Check sheet for the modelled part. Datum: model origin and axes. Units: mm. A direction names the side the tool comes from. Coordinates: 2 decimals unless noted, no trailing zeros. Write each loop counter-clockwise with the first axis right and the second up, starting at its lowest first coordinate (ties: lowest second). Pieces come first, ordered by that corner, then holes. Notation, with made-up numbers: (79.25, -1.75) - (113.25, -1.75) arc R8 ccw to (113.25, 6.25) - close; hole circle Ø9 at (-36.75, 3.5). An arc over 180 degrees is marked (long way). Answer as CSV lines item,"result". Start each with the question number.
Autodesk Inventor part; units mm, degrees
ref_plane "YZ Plane" through (0, 0, 0) normal (1, 0, 0) x (0, 1, 0)
ref_plane "XZ Plane" through (0, 0, 0) normal (0, 1, 0) x (-1, 0, 0)
ref_plane "XY Plane" through (0, 0, 0) normal (0, 0, 1) x (1, 0, 0)
sketch "Sketch4" plane through (0, 0, 0) normal (0, 1, 0) x (-1, 0, 0)
  line L0 (20, -35) -> (-20, -35)
  line L1 (-20, -35) -> (-20, 0)
  line L2 (-20, 0) -> (20, 0)
  line L3 (20, 0) -> (20, -35)
  point P0 (0, 0)
  point P1 (0, 0)
  dimension "d36" = 40
  dimension "d37" = 35
extrude "Plate2" add sketch "Sketch4" along normal blind 3
sketch "Sketch5" plane through (0, 0, 0) normal (0, -1, 0) x (1, 0, 0)
  circle A0 centre (0, -20) radius 6.5
  line L0 (0, 0) -> (0, -35) construction
  line L1 (20, -35) -> (-20, -35) construction
  dimension "d40" = 15
  dimension "d41" = 13
extrude "Cut1" cut sketch "Sketch5" against normal blind 3
sketch "Sketch6" plane through (-20, 3, -3) normal (0, 0, 1) x (1, 0, 0)
  line L0 (40, 0) -> (0, 0)
  line L1 (0, 0) -> (0, -40)
  line L2 (0, -40) -> (40, -40)
  line L3 (40, -40) -> (40, 0)
edge flange "Flange1" height 40 angle 90 thickness 3 bend radius 5 thickness toward (0, 0, 1) relief round relief width 3 relief depth 1.5 edges at (0, 0, 0) wall of the first edge with corners at (20, 3, -3) (-20, 3, -3) (-20, -37, -3) (20, -37, -3)
bend "Bend1"
corner "Corner1"
fillet "Corner Round6" radius 6 4 edges at (20, -37, -1.5) (-20, 1.5, -35) (20, 1.5, -35) (-20, -37, -1.5)
equation "\"d42\" = Thickness"
equation "\"d38\" = Thickness"
equation "\"d44\" = BendReliefWidth"
equation "\"d45\" = BendReliefDepth"
equation "\"d46\" = MinimumRemnant"
equation "\"d47\" = TransitionRadius"
equation "\"d50\" = BendRadius"
equation "\"d51\" = CornerReliefSize"
equation "\"d52\" = GapSize"
equation "\"d53\" = JacobiRadiusSize"
equation "\"BendReliefWidth\" = Thickness"
equation "\"BendReliefDepth\" = 0.5 * Thickness"
equation "\"CornerReliefSize\" = 4 * Thickness"
equation "\"MinimumRemnant\" = 2 * Thickness"
equation "\"TransitionRadius\" = BendRadius"
equation "\"JacobiRadiusSize\" = BendRadius"
equation "\"GapSize\" = Thickness"
properties part number "NDM-VOS 913 flange bolt" material "Stainless Steel"
(1) Release check for a two-part mould opening along X. For faces 1 (the face through (-0.846, 1.479, -13.555)), 2 (the face through (-18.289, -35.196, -1.479)), 3 (the face through (0, -21, -3)) record: pulls with the +X half, pulls with the -X half, needs draft (parallel to the pull), parting line crosses it, or undercut.
(2) Material ranges on probe 1 along Z at (x, y) = (-9.5, -32.5); probe 2 along Y at (x, z) = (14, -14); probe 3 along Z at (x, y) = (0, 1.1), recorded low to high. Write a range as from..to.
(3) Go/stop test with flat-tipped pins: P1, Ø13.5, axis at x = -1.5, z = -16.5, coming from the -Y side; P2, Ø11.5, axis at x = 0, z = -20, coming from the +Y side; P3, Ø1, axis at x = -15.5, y = -13, coming from the -Z side. Record where each tip stops, or that it passes through.
(4) Cross-section at A-A on z = -20. Record the boundary of the cut face in (x, y), plus the area to 3 significant figures.
(5) Cross-section at B-B on x = 0. Record the boundary of the cut face in (y, z), plus the area to 3 significant figures.
(6) Tool access check on faces 4 (the face through (0, 0, -27)), 5 (the face through (18.289, 1.521, -33.196)). Record the directions out of +Z, -Z, +X, -X, +Y, -Y that give a thin tool (end or side, any length) a straight path to the whole face; none if there is none.
(7) Cross-section at C-C on x = 9.5. Record the boundary of the cut face in (y, z).
(8) Cross-section at D-D on y = -13. Record the boundary of the cut face in (x, z).
Checked values:
1,face 1,"undercut"
1,face 2,"pulls with the -X half"
1,face 3,"needs draft"
2,probe 1,"-3..0"
2,probe 2,"0..3"
2,probe 3,"-35..-26.5, -13.5..-2.82"
3,P1,"y = 0"
3,P2,"through"
3,P3,"z = -3"
4,outline,"(-20, 0) - (-6.5, 0) - (-6.5, 3) - (-20, 3) - close; (6.5, 0) - (20, 0) - (20, 3) - (6.5, 3) - close"
4,area,"81.0 mm^2"
5,outline,"(-37, -3) - (-5, -3) arc R5 cw to (0, -8) - (0, -13.5) - (3, -13.5) - (3, -8) arc R8 ccw to (-5, 0) - (-37, 0) - close; (0, -35) - (3, -35) - (3, -26.5) - (0, -26.5) - close"
5,area,"169 mm^2"
6,face 4,"-Z, +X, -X, -Y"
6,face 5,"-Z, +X, +Y, -Y"
7,outline,"(-37, -3) - (-5, -3) arc R5 cw to (0, -8) - (0, -35) - (3, -35) - (3, -8) arc R8 ccw to (-5, 0) - (-37, 0) - close"
8,outline,"(-20, -3) - (20, -3) - (20, 0) - (-20, 0) - close"
